Geometry check sheet. Reference: the model listing, model coordinates, mm. Coordinates: 2 decimals unless noted, no trailing zeros. Order: outer loops, then holes, each group sorted by start corner. A loop starts at its lowest first (then second) coordinate and runs counter-clockwise, first axis right, second up. Notation, with made-up numbers: (-0.5, -11) - (23.5, -11) arc R14 ccw to (23.5, -7) - close; hole circle Ø1 at (40, -19). An arc over 180 degrees is marked (long way). Use CSV: the item, a comma, the result in double quotes. Start each with the question number.
1) Sectioned sample at B-B, the plane z = -5.5. Record the cut outline in (x, y), and give its area (3 significant figures).
2) Thickness scan on probe 1 along Y at (x, z) = (24, 5.25); probe 2 along Z at (x, y) = (70, -9.3). Record the ranges inside material, lowest first. Write a range as [from, to].
3) Sectioned sample at A-A, the plane y = 5. Record the cut outline in (x, z).
4) Sectioned sample at C-C, the plane x = 153. Record the cut outline in (y, z), and give its area (3 significant figures).
5) Depth check by flat-ended pin: P1, Ø5, axis at x = -70, z = 0, coming from the +Y side; P2, Ø5, axis at y = -5, z = -5, coming from the -X side. Enter the tip coordinate at first touch or a pass-through.
from build123d import *

# Parameters (mm, degrees)
SKETCH_1_W               = 20
SKETCH_1_H               = 20
SKETCH_1_W_2             = 17.6
SKETCH_1_H_2             = 17.6
EXTRUDE_2_DEPTH          = 280
CUT_EXTRUDE_2_DEPTH      = 281.356915378
CUT_EXTRUDE_2_DEPTH_BACK = 281.356915378
SKETCH_4_W               = 20
SKETCH_4_H               = 10
CUT_EXTRUDE_3_DEPTH      = 281.891438104
CUT_EXTRUDE_3_DEPTH_BACK = 281.891438104
SKETCH_5_R               = 1.6


with BuildPart() as part:
    # 草图1 → 凸台-拉伸2 (new, symmetric)
    with BuildSketch(Plane(origin=(0, 0, 0), x_dir=(0, 0, -1), z_dir=(1, 0, 0))):
        Rectangle(SKETCH_1_W, SKETCH_1_H)
        Rectangle(SKETCH_1_W_2, SKETCH_1_H_2, mode=Mode.SUBTRACT)
    extrude(amount=EXTRUDE_2_DEPTH, both=True)

    # 草图4 → 切除-拉伸2 (cut, two sides: drawn at the far end of the back side and taken through both)
    with BuildSketch(Plane.XY.offset(-CUT_EXTRUDE_2_DEPTH_BACK)):
        with Locations((85, -5)):
            Rectangle(SKETCH_4_W, SKETCH_4_H)
        with Locations((-85, -5)):
            Rectangle(SKETCH_4_W, SKETCH_4_H)
    extrude(amount=CUT_EXTRUDE_2_DEPTH + CUT_EXTRUDE_2_DEPTH_BACK, mode=Mode.SUBTRACT)

    # 草图5 → 切除-拉伸3 (cut, two sides: drawn at the far end of the back side and taken through both)
    with BuildSketch(Plane(origin=(0, 10, 0), x_dir=(1, 0, 0), z_dir=(0, 1, 0)).offset(-CUT_EXTRUDE_3_DEPTH_BACK)):
        with Locations(Location((115, 0, 0), (0, 0, 270))):
            Circle(SKETCH_5_R)
        with Locations(Location((165, 0, 0), (0, 0, 270))):
            Circle(SKETCH_5_R)
        with Locations(Location((265, 0, 0), (0, 0, 270))):
            Circle(SKETCH_5_R)
        with Locations(Location((215, 0, 0), (0, 0, 270))):
            Circle(SKETCH_5_R)
        with Locations(Location((-215, 0, 0), (0, 0, 90))):
            Circle(SKETCH_5_R)
        with Locations(Location((-265, 0, 0), (0, 0, 90))):
            Circle(SKETCH_5_R)
        with Locations(Location((-165, 0, 0), (0, 0, 90))):
            Circle(SKETCH_5_R)
        with Locations(Location((-115, 0, 0), (0, 0, 90))):
            Circle(SKETCH_5_R)
        with Locations(Location((70, 0, 0), (0, 0, 90))):
            Circle(SKETCH_5_R)
        with Locations(Location((-70, 0, 0), (0, 0, 90))):
            Circle(SKETCH_5_R)
        with Locations(Location((40, 0, 0), (0, 0, 90))):
            Circle(SKETCH_5_R)
        with Locations(Location((-40, 0, 0), (0, 0, 90))):
            Circle(SKETCH_5_R)
    extrude(amount=CUT_EXTRUDE_3_DEPTH + CUT_EXTRUDE_3_DEPTH_BACK, mode=Mode.SUBTRACT)


solid = part.part
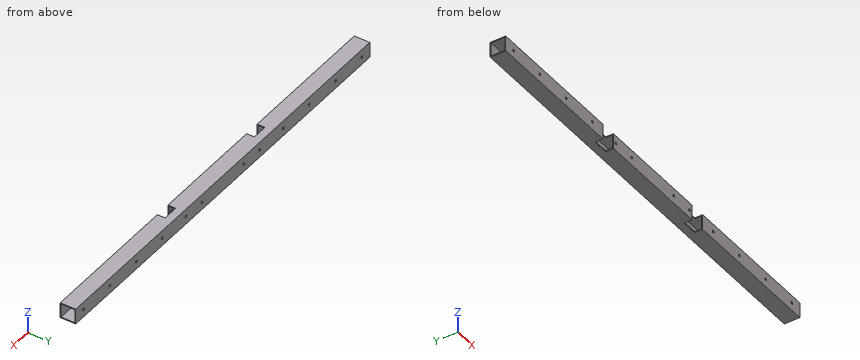
Evaluation:
1,outline,"(-280, -10) - (-95, -10) - (-95, -8.8) - (-280, -8.8) - close; (-280, 8.8) - (280, 8.8) - (280, 10) - (-280, 10) - close; (-75, -10) - (75, -10) - (75, -8.8) - (-75, -8.8) - close; (95, -10) - (280, -10) - (280, -8.8) - (95, -8.8) - close"
1,area,"1,300 mm²"
2,probe 1,"[-10, -8.8], [8.8, 10]"
2,probe 2,"[-10, -1.6], [1.6, 10]"
3,outline,"(-280, -10) - (280, -10) - (280, -8.8) - (-280, -8.8) - close; (-280, 8.8) - (280, 8.8) - (280, 10) - (-280, 10) - close"
4,outline,"(-10, -10) - (10, -10) - (10, 10) - (-10, 10) - close; hole (-8.8, -8.8) - (8.8, -8.8) - (8.8, 8.8) - (-8.8, 8.8) - close"
4,area,"90.2 mm²"
5,P1,"y = 10"
5,P2,"through"
